Can you work these out from the model? Positions are in its coordinate system, mm. Face numbers are marked on the shaded views. A direction names the side the tool comes from. Coordinates: 2 decimals unless noted, no trailing zeros. Write each loop counter-clockwise with the first axis right and the second up, starting at its lowest first coordinate (ties: lowest second). Pieces come first, ordered by that corner, then holes. Notation, with made-up numbers: (11, 5.5) -> (55, 5.5) arc R23 ccw to (55, 20.5) -> close; hole circle Ø4 at (78, 31). An arc over 180 degrees is marked (long way). Answer as CSV lines item,"result". Start each with the question number.
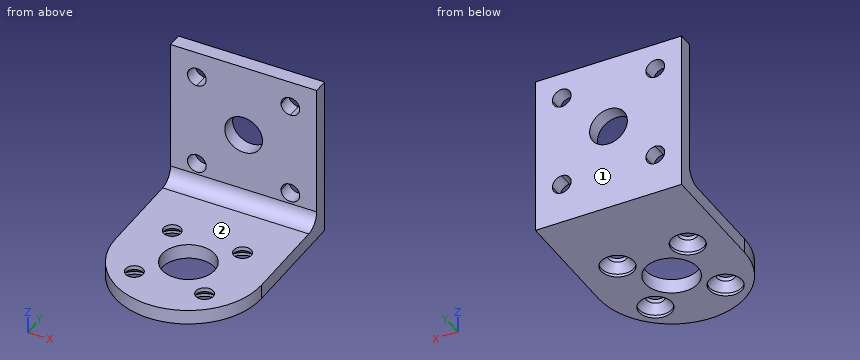
```python
from build123d import *

# Parameters (mm, degrees)
SKETCH1_R           = 2.8
SKETCH1_R_2         = 4.5
BOSS_EXTRUDE1_DEPTH = 2.5
SKETCH2_W           = 25
SKETCH2_H           = 2.5
BOSS_EXTRUDE2_DEPTH = 25
FILLET1_R           = 2.5
SKETCH4_R           = 3.229450522
CUT_EXTRUDE1_DEPTH  = 10
BOSS_EXTRUDE3_START = -2
SKETCH3_R           = 2.8
SKETCH3_R_2         = 1.5
BOSS_EXTRUDE3_DEPTH = 0.5
CHAMFER4_SIZE       = 1.5


with BuildPart() as part:
    # Sketch1 → Boss-Extrude1 (new body)
    with BuildSketch(Plane.XY):
        with BuildLine():
            Line((-12.5, 0), (-12.5, 20))
            Line((-12.5, 20), (12.5, 20))
            Line((12.5, 20), (12.5, 0))
            ThreePointArc((12.5, 0), (0, -12.5), (-12.5, 0))
        make_face()
        with Locations((-6.01040764, 6.01040764)):
            Circle(SKETCH1_R, mode=Mode.SUBTRACT)
        with Locations((-6.01040764, -6.01040764)):
            Circle(SKETCH1_R, mode=Mode.SUBTRACT)
        with Locations((6.01040764, -6.01040764)):
            Circle(SKETCH1_R, mode=Mode.SUBTRACT)
        with Locations((6.01040764, 6.01040764)):
            Circle(SKETCH1_R, mode=Mode.SUBTRACT)
        Circle(SKETCH1_R_2, mode=Mode.SUBTRACT)
    extrude(amount=BOSS_EXTRUDE1_DEPTH)

    # Sketch2 → Boss-Extrude2 (add)
    with BuildSketch(Plane.XY.offset(2.5)):
        with Locations((0, 18.75)):
            Rectangle(SKETCH2_W, SKETCH2_H)
    extrude(amount=BOSS_EXTRUDE2_DEPTH)

    # Fillet1
    fillet1_edges = [part.edges().sort_by_distance(p)[0] for p in [
        (0, 17.5, 2.5),
    ]]
    fillet(fillet1_edges, radius=FILLET1_R)

    # Sketch4 → Cut-Extrude1 (cut)
    with BuildSketch(Plane(origin=(0, 20, 0), x_dir=(1, 0, 0), z_dir=(0, 1, 0))):
        with BuildLine():
            ThreePointArc((-8, -21.4), (-9.13137085, -24.13137085), (-6.4, -23))
            Line((-6.4, -23), (-8, -23))
            Line((-8, -23), (-8, -21.4))
        make_face()
        with BuildLine():
            Line((-8, -23), (-6.4, -23))
            ThreePointArc((-6.4, -23), (-6.86862915, -21.86862915), (-8, -21.4))
            Line((-8, -21.4), (-8, -23))
        make_face()
        with BuildLine():
            ThreePointArc((8, -21.4), (6.86862915, -21.86862915), (6.4, -23))
            Line((6.4, -23), (8, -23))
            Line((8, -23), (8, -21.4))
        make_face()
        with BuildLine():
            Line((8, -23), (6.4, -23))
            ThreePointArc((6.4, -23), (8, -24.6), (9.6, -23))
            ThreePointArc((9.6, -23), (9.13137085, -21.86862915), (8, -21.4))
            Line((8, -21.4), (8, -23))
        make_face()
        with BuildLine():
            ThreePointArc((6.4, -7), (6.86862915, -8.13137085), (8, -8.6))
            Line((8, -8.6), (8, -7))
            Line((8, -7), (6.4, -7))
        make_face()
        with BuildLine():
            Line((8, -7), (8, -8.6))
            ThreePointArc((8, -8.6), (9.13137085, -8.13137085), (9.6, -7))
            ThreePointArc((9.6, -7), (8, -5.4), (6.4, -7))
            Line((6.4, -7), (8, -7))
        make_face()
        with Locations(Location((0, -15, 0), (0, 0, 270))):
            Circle(SKETCH4_R)
        with BuildLine():
            ThreePointArc((-6.4, -7), (-9.13137085, -5.86862915), (-8, -8.6))
            Line((-8, -8.6), (-8, -7))
            Line((-8, -7), (-6.4, -7))
        make_face()
        with BuildLine():
            Line((-8, -7), (-8, -8.6))
            ThreePointArc((-8, -8.6), (-6.86862915, -8.13137085), (-6.4, -7))
            Line((-6.4, -7), (-8, -7))
        make_face()
    extrude(amount=-CUT_EXTRUDE1_DEPTH, mode=Mode.SUBTRACT)

    # Sketch3 → Boss-Extrude3 (add)
    # profile 1 of 4: a face of its own
    with BuildSketch(Plane(origin=(0, 0, 0), x_dir=(-1, 0, 0), z_dir=(0, 0, -1)).offset(BOSS_EXTRUDE3_START)):
        with Locations(Location((-6.01040764, 6.01040764, 0), (0, 0, 180))):
            Circle(SKETCH3_R)
        with Locations(Location((-6.01040764, 6.01040764, 0), (0, 0, 180))):
            Circle(SKETCH3_R_2, mode=Mode.SUBTRACT)
    # profile 2 of 4: a face of its own
    with BuildSketch(Plane(origin=(0, 0, 0), x_dir=(-1, 0, 0), z_dir=(0, 0, -1)).offset(BOSS_EXTRUDE3_START)):
        with Locations(Location((6.01040764, 6.01040764, 0), (0, 0, 180))):
            Circle(SKETCH3_R)
        with Locations(Location((6.01040764, 6.01040764, 0), (0, 0, 180))):
            Circle(SKETCH3_R_2, mode=Mode.SUBTRACT)
    # profile 3 of 4: a face of its own
    with BuildSketch(Plane(origin=(0, 0, 0), x_dir=(-1, 0, 0), z_dir=(0, 0, -1)).offset(BOSS_EXTRUDE3_START)):
        with Locations(Location((6.01040764, -6.01040764, 0), (0, 0, 180))):
            Circle(SKETCH3_R)
        with Locations(Location((6.01040764, -6.01040764, 0), (0, 0, 180))):
            Circle(SKETCH3_R_2, mode=Mode.SUBTRACT)
    # profile 4 of 4: a face of its own
    with BuildSketch(Plane(origin=(0, 0, 0), x_dir=(-1, 0, 0), z_dir=(0, 0, -1)).offset(BOSS_EXTRUDE3_START)):
        with Locations(Location((-6.01040764, -6.01040764, 0), (0, 0, 180))):
            Circle(SKETCH3_R)
        with Locations(Location((-6.01040764, -6.01040764, 0), (0, 0, 180))):
            Circle(SKETCH3_R_2, mode=Mode.SUBTRACT)
    extrude(amount=-BOSS_EXTRUDE3_DEPTH)

    # Chamfer4
    # the kernel refuses this chamfer: 1.5 mm, written as the material it adds along each edge
    with BuildSketch(Plane(origin=(6.01040764, 6.01040764, 2), x_dir=(1, 0, 0), z_dir=(0, 1, 0))) as chamfer4_piece_1_section:
        Polygon((2.8, CHAMFER4_SIZE), (2.8 - CHAMFER4_SIZE, 0), (2.8, 0), align=None)
    chamfer4_piece_1 = revolve(axis=Axis((6.01040764, 6.01040764, 2), (0, 0, -1)), mode=Mode.PRIVATE)
    chamfer4_piece_1 = chamfer4_piece_1 - Plane(origin=(6.01040764, 6.01040764, 1.147189391), x_dir=(1, 0, 0), z_dir=(0, 0, -1)) * Cylinder(1.5, 12, mode=Mode.PRIVATE)
    add(chamfer4_piece_1)
    with BuildSketch(Plane(origin=(-6.01040764, -6.01040764, 2), x_dir=(1, 0, 0), z_dir=(0, 1, 0))) as chamfer4_piece_2_section:
        Polygon((2.8, CHAMFER4_SIZE), (2.8 - CHAMFER4_SIZE, 0), (2.8, 0), align=None)
    chamfer4_piece_2 = revolve(axis=Axis((-6.01040764, -6.01040764, 2), (0, 0, -1)), mode=Mode.PRIVATE)
    chamfer4_piece_2 = chamfer4_piece_2 - Plane(origin=(-6.01040764, -6.01040764, 1.147189391), x_dir=(1, 0, 0), z_dir=(0, 0, -1)) * Cylinder(1.5, 12, mode=Mode.PRIVATE)
    add(chamfer4_piece_2)
    with BuildSketch(Plane(origin=(6.01040764, -6.01040764, 2), x_dir=(1, 0, 0), z_dir=(0, 1, 0))) as chamfer4_piece_3_section:
        Polygon((2.8, CHAMFER4_SIZE), (2.8 - CHAMFER4_SIZE, 0), (2.8, 0), align=None)
    chamfer4_piece_3 = revolve(axis=Axis((6.01040764, -6.01040764, 2), (0, 0, -1)), mode=Mode.PRIVATE)
    chamfer4_piece_3 = chamfer4_piece_3 - Plane(origin=(6.01040764, -6.01040764, 1.147189391), x_dir=(1, 0, 0), z_dir=(0, 0, -1)) * Cylinder(1.5, 12, mode=Mode.PRIVATE)
    add(chamfer4_piece_3)
    with BuildSketch(Plane(origin=(-6.01040764, 6.01040764, 2), x_dir=(1, 0, 0), z_dir=(0, 1, 0))) as chamfer4_piece_4_section:
        Polygon((2.8, CHAMFER4_SIZE), (2.8 - CHAMFER4_SIZE, 0), (2.8, 0), align=None)
    chamfer4_piece_4 = revolve(axis=Axis((-6.01040764, 6.01040764, 2), (0, 0, -1)), mode=Mode.PRIVATE)
    chamfer4_piece_4 = chamfer4_piece_4 - Plane(origin=(-6.01040764, 6.01040764, 1.147189391), x_dir=(1, 0, 0), z_dir=(0, 0, -1)) * Cylinder(1.5, 12, mode=Mode.PRIVATE)
    add(chamfer4_piece_4)


solid = part.part
```
Q1. Which directions (+Z, -Z, +X, -X, +Y, -Y) give clear straight access to the entire face, cutting with the end or side of a thin tool? Please do the marked faces 1 and 2.
Q2. I need wall thicknesses on L1, parallel to Z at x = -8, y = 18.45; L2, parallel to Z at x = -5.75, y = -1; L3, parallel to Y at x = 11.5, z = 9.5. Which ranges of each line are inside material? Lowest first, please.
Q3. Imagine slicing it at C-C (y = -7). State how many separate pieces and enclosed holes the cut face has, then the cut area to 3 significant figures.
Q4. For pin 1 (3.5 mm diameter, centred on x = 6.01, y = 6.01, fed in from -Z); pin 2 (5 mm diameter, centred on x = 6.01, y = -6.01, fed in from -Z); pin 3 (6.5 mm diameter, centred on x = -6.01, y = 6.01, fed in from +Z), each with a flat end and sliding along its axis, tell me the tip position at first contact or that it passes through.
Q5. Imagine slicing it at B-B (x = 0). Write out the boundary of the cut face in (y, z).
Q6. Imagine slicing it at A-A (z = 15). Write out the boundary of the cut face in (x, y), then the cut area to 3 significant figures.
Entries:
1,face 1,"+Z, -Z, +X, -X, +Y"
1,face 2,"+Z, +X, -X, -Y"
2,L1,"0 to 5.4, 8.6 to 21.4, 24.6 to 27.5"
2,L2,"0 to 2.5"
2,L3,"17.5 to 20"
3,separate pieces,"3"
3,enclosed holes,"0"
3,area,"33.5 mm2"
4,pin 1,"z = 1.55"
4,pin 2,"z = 0.8"
4,pin 3,"z = 2.5"
5,outline,"(-12.5, 0) -> (-4.5, 0) -> (-4.5, 2.5) -> (-12.5, 2.5) -> close; (4.5, 0) -> (20, 0) -> (20, 11.77) -> (17.5, 11.77) -> (17.5, 5) arc R2.5 cw to (15, 2.5) -> (4.5, 2.5) -> close; (17.5, 18.23) -> (20, 18.23) -> (20, 27.5) -> (17.5, 27.5) -> close"
6,outline,"(-12.5, 17.5) -> (-3.23, 17.5) -> (-3.23, 20) -> (-12.5, 20) -> close; (3.23, 17.5) -> (12.5, 17.5) -> (12.5, 20) -> (3.23, 20) -> close"
6,area,"46.4 mm2"
